Verification items for the finished model (mm, model axes). Face numbers are marked on the shaded views. A direction names the side the tool comes from. Coordinates: 2 decimals unless noted, no trailing zeros. Loops run counter-clockwise (first coordinate to the right, second up) from the corner with the lowest first, then second, coordinate; pieces in that order, holes last. Notation, with made-up numbers: (-22.5, -15) -> (27.5, -15) arc R19 cw to (27.5, 3) -> close; hole circle Ø8 at (45.5, -39.5). An arc over 180 degrees is marked (long way). Use CSV: the item, a comma, the result in double quotes. Start each with the question number.
```python
from build123d import *

# Parameters (mm, degrees)
F1_DEPTH  = 16
F2_W      = 70
F2_H      = 3
F3_DEPTH  = 2
F4_W      = 50
F4_H      = 12
F5_DEPTH  = 2
F6_R      = 1
F9_DEPTH  = 2
F11_DEPTH = 38.001
F13_D     = 4
F14_R     = 3
F14_R_2   = 2
F15_DEPTH = 5
F16_R     = 3


# Not quite as in the source:
# - a pattern or mirror of a feature is missing from the dataset's text; its kind, count and spacing are read off the source's solid


with BuildPart() as f1:
    # F0 (on Front) → F1 (new body)
    with BuildSketch(Plane.XZ):
        with BuildLine():
            Line((94, 11), (0, 11))
            ThreePointArc((0, 11), (-11, 0), (0, -11))
            Line((0, -11), (19, -11))
            ThreePointArc((19, -11), (21.7681124643, -11.8361612201), (23.6103896104, -14.064978646))
            ThreePointArc((23.6103896104, -14.064978646), (47.8232093534, -44.5540629158), (84.3688749643, -57.9801280344))
            ThreePointArc((84.3688749643, -57.9801280344), (88.282737688, -59.7162176184), (91.4888593469, -62.5540182408))
            Line((91.4888593469, -62.5540182408), (92.7928354795, -61))
            ThreePointArc((92.7928354795, -61), (89.1281978331, -57.8850966861), (84.7034264019, -56))
            ThreePointArc((84.7034264019, -56), (49.0672193413, -42.9854179344), (25.4545454545, -13.2909701044))
            ThreePointArc((25.4545454545, -13.2909701044), (22.87535745, -10.1706257081), (19, -9))
            Line((19, -9), (0, -9))
            ThreePointArc((0, -9), (-9, 0), (0, 9))
            Line((0, 9), (94, 9))
            Line((94, 9), (94, 11))
        make_face()
    extrude(amount=F1_DEPTH)

    # F2 (on face) → F3 (join)
    with BuildSketch(Plane.XY.offset(11)):
        with Locations((59, -17.5)):
            Rectangle(F2_W, F2_H)
    extrude(amount=-F3_DEPTH)

    # F4 (on face) → F5 (join)
    with BuildSketch(Plane.XZ.offset(19)):
        with Locations((69, 3)):
            Rectangle(F4_W, F4_H)
    extrude(amount=-F5_DEPTH)

    # F6
    f6_edges = [f1.edges().sort_by_distance(p)[0] for p in [
        (59, -19, 11),
    ]]
    fillet(f6_edges, radius=F6_R)

    # F7: F1 across plane


with BuildPart() as f1_1:
    add(f1.part)
    add(f1.part.mirror(Plane.XZ))

    # F8 (on face) → F9 (cut)
    with BuildSketch(Plane.XY.offset(11)):
        with BuildLine():
            Line((94, 12), (34, 12))
            ThreePointArc((34, 12), (22, 0), (34, -12))
            Line((34, -12), (94, -12))
            Line((94, -12), (94, 12))
        make_face()
    extrude(amount=-F9_DEPTH, mode=Mode.SUBTRACT)

    # F10 (on face) → F11 (cut, through all)
    with BuildSketch(Plane.XZ.offset(19)):
        with BuildLine():
            ThreePointArc((50, 5), (47, 2), (50, -1))
            Line((50, -1), (70, -1))
            ThreePointArc((70, -1), (73, 2), (70, 5))
            Line((70, 5), (50, 5))
        make_face()
    extrude(amount=-F11_DEPTH, mode=Mode.SUBTRACT)

    # F13 (through all)
    with Locations(Plane.XZ.offset(19)):
        with Locations((80, 3)):
            Hole(F13_D / 2)

    # F14 (on face) → F15 (join)
    with BuildSketch(Plane(origin=(0, -17, 0), x_dir=(-1, 0, 0), z_dir=(0, 1, 0))):
        with Locations((-80, 3)):
            Circle(F14_R)
        with Locations((-80, 3)):
            Circle(F14_R_2, mode=Mode.SUBTRACT)
    f15 = extrude(amount=F15_DEPTH)

    # F15_copies: F15 across plane
    add(f15.mirror(Plane.ZX))

    # F16
    f16_edges = [f1_1.edges().sort_by_distance(p)[0] for p in [
        (94, 18, -3),
        (44, 18, -3),
        (94, -18, -3),
        (44, -18, -3),
    ]]
    fillet(f16_edges, radius=F16_R)


solid = f1_1.part
```
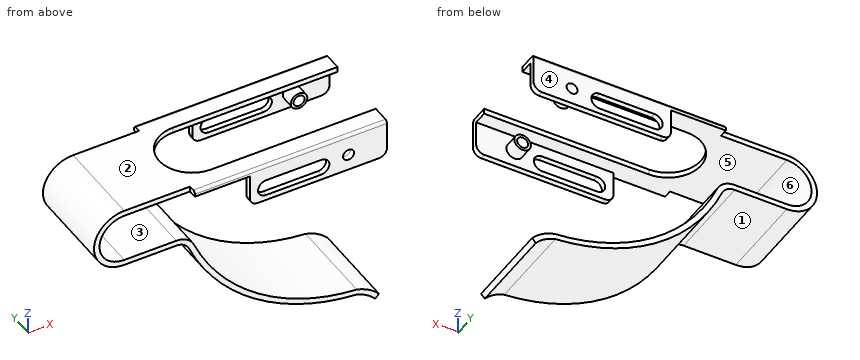
1. Set-up check for the marked faces 1, 2 and 3: record each of +Z, -Z, +X, -X, +Y, -Y from which the full face is reachable in a straight line by a thin tool's end or side.
2. Release check for a two-part mould opening along Y. For the marked faces 4, 5 and 6 record: released by +Y, released by -Y, zero draft, split by the parting line, or undercut.
3. Cross-section at C-C, the plane y = 8. Record the boundary of the cut face in (x, z).
4. Cross-section at A-A, the plane x = 11. Record the boundary of the cut face in (y, z).
5. Depth check by flat-ended pin: pin 1 (3 mm diameter, centred on x = 80, z = 3, fed in from +Y); pin 2 (21 mm diameter, centred on x = 9.5, y = -4.5, fed in from -Z); pin 3 (5 mm diameter, centred on x = 37.5, y = -14.5, fed in from -Z); pin 4 (4 mm diameter, centred on y = -1, z = -33, fed in from +X). Enter the tip coordinate at first touch or a pass-through.
6. Cross-section at B-B, the plane x = 80. State how many separate pieces and enclosed holes the cut face has, plus the area to 3 significant figures.
7. Scan lines: line 1 (Z direction, x = 7, y = 2.5); line 2 (Z direction, x = 80, y = -17.55); line 3 (Z direction, x = 80, y = -14). Record each from-to range of solid material in increasing order.
Solution:
1,face 1,"-Z, -X, +Y, -Y"
1,face 2,"+Z, +X, -X, +Y, -Y"
1,face 3,"+X, +Y, -Y"
2,face 4,"released by +Y"
2,face 5,"undercut"
2,face 6,"zero draft"
3,outline,"(0, -11) -> (19, -11) arc R5 cw to (23.61, -14.06) arc R72 ccw to (84.37, -57.98) arc R14 cw to (91.49, -62.55) -> (92.79, -61) arc R16 ccw to (84.7, -56) arc R70 cw to (25.45, -13.29) arc R7 ccw to (19, -9) -> (0, -9) arc R9 cw to (0, 9) -> (25.06, 9) -> (25.06, 11) -> (0, 11) arc R11 ccw to start"
4,outline,"(-16, -11) -> (16, -11) -> (16, -9) -> (-16, -9) -> close; (-16, 9) -> (16, 9) -> (16, 11) -> (-16, 11) -> close"
5,pin 1,"passes through"
5,pin 2,"stops at z = -11.1"
5,pin 3,"stops at z = -38.01"
5,pin 4,"stops at x = 39.81"
6,separate pieces,"5"
6,enclosed holes,"0"
6,area,"144 mm2"
7,line 1,"z = -11 to -9, 9 to 11"
7,line 2,"z = -3 to 1, 5 to 11"
7,line 3,"z = -57.5 to -55.48, 0 to 1, 5 to 6, 9 to 11"
